Read the model definition and answer for the solid it produces. Units are mm, in the model's axes. Face numbers are marked on the shaded views. A direction names the side the tool comes from. Give positions to 0.01 mm unless a question says otherwise; leave off trailing zeros. Order: outer loops, then holes, each group sorted by start corner. A loop starts at its lowest first (then second) coordinate and runs counter-clockwise, first axis right, second up.
```python
from build123d import *

# Parameters (mm, degrees)
EXTRUDE_1_DEPTH = 20
SKETCH_2_W      = 20
SKETCH_2_H      = 15
SKETCH_2_R      = 2.75
EXTRUDE_2_DEPTH = 5
FILLET_1_R      = 2


with BuildPart() as part:
    # 草图1 → 凸台-拉伸1 (new body)
    with BuildSketch(Plane(origin=(0, 0, 0), x_dir=(0, 0, -1), z_dir=(1, 0, 0))):
        Polygon((-38.386760485, 40.8), (-38.386760485, 0), (34.113239515, 0), (34.113239515, 20.4), align=None)
    extrude(amount=EXTRUDE_1_DEPTH)

    # 草图2 → 凸台-拉伸2 (add)
    # profile 1 of 2: a face of its own
    with BuildSketch(Plane.XZ):
        with Locations((10, 45.886760485)):
            Rectangle(SKETCH_2_W, SKETCH_2_H)
        with Locations(Location((10, 45.886760485, 0), (0, 0, 90))):
            Circle(SKETCH_2_R, mode=Mode.SUBTRACT)
    # profile 2 of 2: a face of its own
    with BuildSketch(Plane.XZ):
        with Locations((10, -41.613239515)):
            Rectangle(SKETCH_2_W, SKETCH_2_H)
        with Locations(Location((10, -41.613239515, 0), (0, 0, 270))):
            Circle(SKETCH_2_R, mode=Mode.SUBTRACT)
    extrude(amount=-EXTRUDE_2_DEPTH)

    # 圆角1
    fillet_1_edges = [part.edges().sort_by_distance(p)[0] for p in [
        (10, 5, 53.386760485),
        (10, 5, -49.113239515),
        (10, 20.4, -34.113239515),
        (10, 40.8, 38.386760485),
    ]]
    fillet(fillet_1_edges, radius=FILLET_1_R)


solid = part.part
```
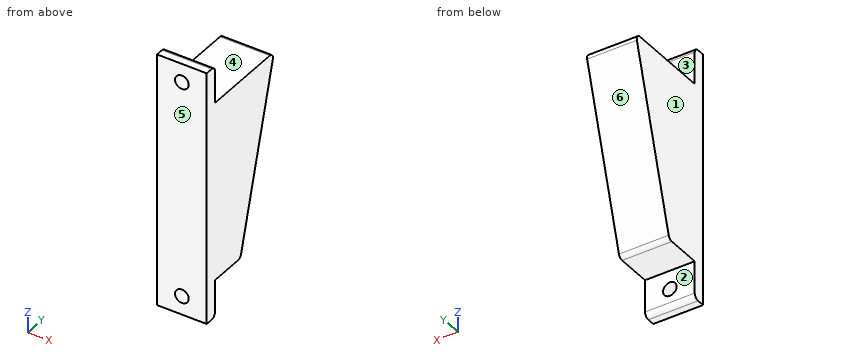
1) The part is cut by section B-B on x = 6. Determine the outline of the cut face in (y, z).
Final values:
outline: (0, -49.11) - (3, -49.11) arc R2 ccw to (5, -47.11) - (5, -34.11) - (18.89, -34.11) arc R2 ccw to (20.81, -32.65) - (40.08, 35.85) arc R2 ccw to (38.16, 38.39) - (5, 38.39) - (5, 51.39) arc R2 ccw to (3, 53.39) - (0, 53.39) - close
2) Given pin 1 (6.5 mm diameter, centred on x = 10, z = -41.61, fed in from +Y); pin 2 (10 mm diameter, centred on x = 15.5, y = 17, fed in from -Z); pin 3 (8 mm diameter, centred on x = 17.5, y = 10, fed in from +Z), each flat-ended and moving along its own axis, determine where each tip first touches the part or whether it passes through.
Final values:
pin 1: stops at y = 5
pin 2: stops at z = -34.11
pin 3: stops at z = 38.39
3) A tool of negligible diameter and unlimited length cuts with its end or side. For the marked faces 1, 2 and 3, from which of +Z, -Z, +X, -X, +Y, -Y can it reach the whole face along a straight path? Write none if from no direction.
Final values:
face 1: +Z, -Z, -X, +Y, -Y
face 2: -Z, +X, -X, +Y
face 3: +Z, +X, -X, +Y
4) Consider L1, parallel to Y at x = 5.5, z = -41.5; L2, parallel to Z at x = 2, y = 17; L3, parallel to Y at x = 3.75, z = 1. Determine where each line is inside the solid, lowest interval first.
Final values:
L1: y = 0 to 5
L2: z = -34.11 to 38.39
L3: y = 0 to 30.28
5) The part is cut by section A-A on x = 10. Determine the outline of the cut face in (y, z).
Final values:
outline: (0, -49.11) - (3, -49.11) arc R2 ccw to (5, -47.11) - (5, -44.36) - (0, -44.36) - close; (0, -38.86) - (5, -38.86) - (5, -34.11) - (18.89, -34.11) arc R2 ccw to (20.81, -32.65) - (40.08, 35.85) arc R2 ccw to (38.16, 38.39) - (5, 38.39) - (5, 43.14) - (0, 43.14) - close; (0, 48.64) - (5, 48.64) - (5, 51.39) arc R2 ccw to (3, 53.39) - (0, 53.39) - close
6) The part is cut by section C-C on y = 7.5. Determine the outline of the cut face in (x, z).
Final values:
outline: (0, -34.11) - (20, -34.11) - (20, 38.39) - (0, 38.39) - close
7) For a pull along Z with two mould halves and no side action, classify the marked faces 4, 5 and 6 as released by +Z, released by -Z, zero draft, split by the parting line, or undercut.
Final values:
face 4: released by +Z
face 5: zero draft
face 6: released by -Z
8) The part is cut by section D-D on z = 20. Determine the outline of the cut face in (x, y), and give its area (3 significant figures).
Final values:
outline: (0, 0) - (20, 0) - (20, 35.63) - (0, 35.63) - close
area: 713 mm2
